The model under review builds one solid part; all positions refer to its coordinate system, in mm. A direction names the side the tool comes from. Give positions to 0.01 mm unless a question says otherwise; leave off trailing zeros. Loops run counter-clockwise (first coordinate to the right, second up) from the corner with the lowest first, then second, coordinate; pieces in that order, holes last. Notation, with made-up numbers: M 57.5,61.5 L 105.5,61.5 A30 ccw 105.5,89.5 Z; hole C 17,60 d8. An arc over 180 degrees is marked long. Return JSON: item names as keys, results as strings.
```python
from build123d import *

# Parameters (mm, degrees)
F1_DEPTH = 5
F3_DEPTH = 240


with BuildPart() as f1:
    # F0 (on Front) → F1 (new body, symmetric)
    with BuildSketch(Plane.XZ):
        with BuildLine():
            Line((14, -105), (14, 105))
            ThreePointArc((14, 105), (0, 119), (-14, 105))
            Line((-14, 105), (-14, -105))
            ThreePointArc((-14, -105), (0, -119), (14, -105))
        make_face()
        with BuildLine():
            ThreePointArc((-6, 105), (0, 111), (6, 105))
            Line((6, 105), (6, -105))
            ThreePointArc((6, -105), (0, -111), (-6, -105))
            Line((-6, -105), (-6, 105))
        make_face(mode=Mode.SUBTRACT)
    extrude(amount=F1_DEPTH, both=True)

    # F2 (on face) → F3 (join)
    with BuildSketch(Plane.YZ.offset(14)):
        with BuildLine():
            ThreePointArc((-5, 0), (0, -5), (5, 0))
            ThreePointArc((5, 0), (0, 5), (-5, 0))
        make_face()
    extrude(amount=F3_DEPTH)


solid = f1.part
```
1) The part is to be moulded in two halves that separate along X. For faces 1 (the face through (0, 0, 111)), 2 (the face through (0, 0, -111)), 3 (the face through (132, -4, -3)), 4 (the face through (14, 0, -53)), say which applies: released by +X, released by -X, zero draft, split by the parting line, or undercut.
From the geometry:
{"face 1": "undercut", "face 2": "undercut", "face 3": "zero draft", "face 4": "released by +X"}
2) Insertion check: pin 1 (6 mm diameter, centred on x = 134, y = -1, fed in from -Z); pin 2 (3 mm diameter, centred on y = -0.5, z = -33, fed in from +X); pin 3 (4 mm diameter, centred on x = 174, y = -2, fed in from +Z). Each pin has a flat end and moves straight along its axis. Give the tip position at first contact, or say it passes through.
From the geometry:
{"pin 1": "z = -5", "pin 2": "x = 14", "pin 3": "z = 5"}
3) Consider section C-C on x = 133. Write out the cut boundary in (y, z), then the cut area to 3 significant figures.
From the geometry:
{"outline": "C 0,0 d10", "area": "78.5 mm²"}
4) Wall thickness on L1, parallel to X at y = -1.5, z = -80; L2, parallel to Z at x = 157.5, y = 0.5; L3, parallel to Z at x = 230, y = -0.75: over which ranges is each line inside the solid? List them lowest first. Write a range as from..to.
From the geometry:
{"L1": "-14..-6, 6..14", "L2": "-4.97..4.97", "L3": "-4.94..4.94"}
5) Consider section A-A on z = 58. Write out the cut boundary in (x, y).
From the geometry:
{"outline": "M -14,-5 L -6,-5 L -6,5 L -14,5 Z; M 6,-5 L 14,-5 L 14,5 L 6,5 Z"}
6) Tool access review of faces 5 (the face through (0, 0, 119)), 6 (the face through (-6, 0, -1)): name each direction out of +Z, -Z, +X, -X, +Y, -Y from which nothing blocks a thin tool from reaching the whole face with its end or side.
From the geometry:
{"face 5": "+Z, +Y, -Y", "face 6": "+Y, -Y"}
7) Consider section B-B on y = -3. Write out the cut boundary in (x, z).
From the geometry:
{"outline": "M -14,-105 A14 ccw 14,-105 L 14,-4 L 254,-4 L 254,4 L 14,4 L 14,105 A14 ccw -14,105 Z; hole M -6,-105 A6 ccw 6,-105 L 6,105 A6 ccw -6,105 Z"}
